Design review of the part built by this model. Coordinates are the model's own, in mm. Face numbers are marked on the shaded views. A direction names the side the tool comes from. Give positions to 0.01 mm unless a question says otherwise; leave off trailing zeros. Loops run counter-clockwise (first coordinate to the right, second up) from the corner with the lowest first, then second, coordinate; pieces in that order, holes last. Notation, with made-up numbers: (41.5, -4.5) -> (59.5, -4.5) arc R33 cw to (59.5, 27.5) -> close; hole circle Ø2 at (59, 41.5). An arc over 180 degrees is marked (long way). Answer in a Markdown table with one row per item. Add a question column.
(1) Draft analysis for pull direction X (two halves, no side actions). For the marked faces 4, 5 and 6, state which applies: +X half, -X half, draft (parallel to the pull), parting line (faces both ways), or undercut.
(2) For pin 1 (0.8 mm diameter, centred on y = -1, z = -1.5, fed in from +X), flat-tipped, find the tip position at first contact; note if it passes through.
(3) Consider section D-D on z = -2. Write out the cut boundary in (x, y), then the cut area to 3 significant figures.
(4) Consider section B-B on y = -1.15. Write out the cut boundary in (x, z), then the cut area to 3 significant figures.
(5) Consider section A-A on x = -6. Write out the cut boundary in (y, z).
(6) For the marked faces 1, 2 and 3, list the 3-axis set-ups (+Z, -Z, +X, -X, +Y, -Y) from which the entire face can be reached by the end or side of a thin tool; tool diameter is ignored.
(7) Consider section C-C on x = -1.25. Write out the cut boundary in (y, z), then the cut area to 3 significant figures.
(8) For line 1 (Y direction, x = -0.25, z = -1.7); line 2 (X direction, y = -1.4, z = -1.25); line 3 (Z direction, x = -6, y = -1.45), list the stretches that pass through material, from the lowest coordinate up.
from build123d import *

# Parameters (mm, degrees)
F0_R      = 0.5
F1_DEPTH  = 2
F0_R_2    = 0.4
F2_DEPTH  = 0.5
F3_R      = 0.4
F4_DEPTH  = 0.5
F5_D      = 1
F6_DEPTH  = 0.5
F7_DEPTH  = 0.5
F8_R      = 0.3
F9_W      = 2
F9_H      = 0.1
F10_DEPTH = 25
F11_R     = 0.49999


# Not quite as in the source:
# - a fillet or chamfer is up to 0.001 mm smaller than in the source, because OpenCascade refuses the exact size
# - a feature names something its author has since deleted; it is built from what else it names


with BuildPart() as f1:
    # F0 (on Front) → F1 (new body)
    with BuildSketch(Plane.XZ):
        with BuildLine():
            Line((-1.5, -1.2454767711), (-1.5, -0.24940907))
            Line((-1.5, -0.24940907), (-4, -0.24940907))
            ThreePointArc((-4, -0.24940907), (-5, -1.24940907), (-4, -2.24940907))
            Line((-4, -2.24940907), (-1.5, -2.24940907))
            Line((-1.5, -2.24940907), (-1.5, -1.2454767711))
        make_face()
        with BuildLine():
            ThreePointArc((-4, -2.24940907), (-5, -1.24940907), (-4, -0.24940907))
            Line((-4, -0.24940907), (-7, -0.24940907))
            Line((-7, -0.24940907), (-7, -2.24940907))
            Line((-7, -2.24940907), (-4, -2.24940907))
        make_face()
        with Locations((-6, -1.24940907)):
            Circle(F0_R, mode=Mode.SUBTRACT)
        with Locations((-6, -1.24940907)):
            Circle(F0_R)
    extrude(amount=F1_DEPTH)

    # F0 (on Front) → F2 (join)
    with BuildSketch(Plane.XZ):
        with BuildLine():
            Line((-1.5, -1.2454767711), (-1.5, -0.24940907))
            Line((-1.5, -0.24940907), (-4, -0.24940907))
            ThreePointArc((-4, -0.24940907), (-5, -1.24940907), (-4, -2.24940907))
            Line((-4, -2.24940907), (-1.5, -2.24940907))
            Line((-1.5, -2.24940907), (-1.5, -1.2454767711))
        make_face()
        with BuildLine():
            Line((0, -0.24940907), (-1, -0.24940907))
            Line((-1, -0.24940907), (-1, -2.24940907))
            Line((-1, -2.24940907), (0, -2.24940907))
            ThreePointArc((0, -2.24940907), (1, -1.24940907), (0, -0.24940907))
        make_face()
        with Locations((0, -1.24940907)):
            Circle(F0_R_2, mode=Mode.SUBTRACT)
        Polygon((-1, -2.24940907), (-1, -0.24940907), (-1.5, -0.24940907), (-1.5, -1.2454767711), (-1.5, -2.24940907), align=None)
        with Locations((0, -1.24940907)):
            Circle(F0_R_2)
    extrude(amount=-F2_DEPTH)

    # F3 (on face) → F4 (join)
    with BuildSketch(Plane.XZ.offset(2)):
        with BuildLine():
            Line((-1.5, -2.24940907), (-1.5, -0.24940907))
            Line((-1.5, -0.24940907), (-4, -0.24940907))
            ThreePointArc((-4, -0.24940907), (-5, -1.24940907), (-4, -2.24940907))
            Line((-4, -2.24940907), (-1.5, -2.24940907))
        make_face()
        with BuildLine():
            Line((0, -0.24940907), (-1, -0.24940907))
            Line((-1, -0.24940907), (-1.5, -0.24940907))
            Line((-1.5, -0.24940907), (-1.5, -2.24940907))
            Line((-1.5, -2.24940907), (0, -2.24940907))
            ThreePointArc((0, -2.24940907), (1, -1.24940907), (0, -0.24940907))
        make_face()
        with Locations((0, -1.24940907)):
            Circle(F3_R, mode=Mode.SUBTRACT)
        with Locations((0, -1.24940907)):
            Circle(F3_R)
    extrude(amount=F4_DEPTH)

    # F5 (through all)
    with Locations(Plane(origin=(0, 0, 0), x_dir=(1, 0, 0), z_dir=(0, 1, 0))):
        with Locations((-6, 1.24940907)):
            Hole(F5_D / 2)

    # F0 (on Front) → F6 (join)
    with BuildSketch(Plane.XZ):
        with Locations((0, -1.24940907)):
            Circle(F0_R_2)
    extrude(amount=F6_DEPTH)

    # F3 (on face) → F7 (join)
    with BuildSketch(Plane.XZ.offset(2)):
        with Locations((0, -1.24940907)):
            Circle(F3_R)
    extrude(amount=-F7_DEPTH)

    # F8
    f8_edges = [f1.edges().sort_by_distance(p)[0] for p in [
        (-0.4, -0.5, -1.249409),
        (-0.4, -1.5, -1.249409),
    ]]
    fillet(f8_edges, radius=F8_R)

    # F9 (on face) → F10 (cut)
    with BuildSketch(Plane(origin=(0, 0, -2.24940907), x_dir=(1, 0, 0), z_dir=(0, 0, -1))):
        with Locations((-6, 1.95)):
            Rectangle(F9_W, F9_H)
        with Locations((-6, 0.05)):
            Rectangle(F9_W, F9_H)
    extrude(amount=-F10_DEPTH, mode=Mode.SUBTRACT)

    # F11 (radius 0.5 in the source; OpenCascade refuses exactly that, so slightly less here)
    f11_edges = [f1.edges().sort_by_distance(p)[0] for p in [
        (-7, -1.9, -1.249409),
        (-7, -0.1, -1.249409),
        (-1.5, -1, -0.249409),
        (-1.5, -1, -2.249409),
    ]]
    fillet(f11_edges, radius=F11_R)


solid = f1.part
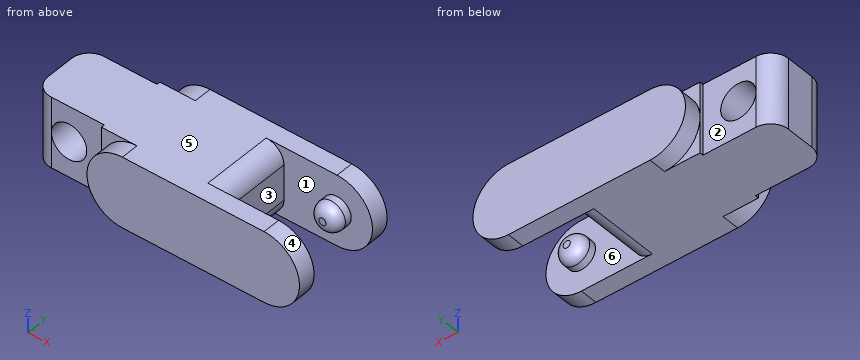
Values follow:
| question | item | result |
|---|---|---|
| 1 | face 4 | +X half |
| 1 | face 5 | draft |
| 1 | face 6 | undercut |
| 2 | pin 1 | x = -1.5 |
| 3 | outline | (-7, -1.4) arc R0.5 ccw to (-6.5, -1.9) -> (-5, -1.9) -> (-5, -2) -> (-4.66, -2) -> (-4.66, -2.5) -> (0.66, -2.5) -> (0.66, -2) -> (-1.57, -2) -> (-1.57, 0) -> (0.66, 0) -> (0.66, 0.5) -> (-4.66, 0.5) -> (-4.66, 0) -> (-5, 0) -> (-5, -0.1) -> (-6.5, -0.1) arc R0.5 ccw to (-7, -0.6) -> close |
| 3 | area | 15.7 mm2 |
| 4 | outline | (-7, -2.25) -> (-2, -2.25) arc R0.5 ccw to (-1.5, -1.75) -> (-1.5, -0.75) arc R0.5 ccw to (-2, -0.25) -> (-7, -0.25) -> close; hole circle Ø1 at (-6, -1.25) |
| 4 | area | 10.1 mm2 |
| 5 | outline | (-1.9, -2.25) -> (-0.1, -2.25) -> (-0.1, -1.75) -> (-1.9, -1.75) -> close; (-1.9, -0.75) -> (-0.1, -0.75) -> (-0.1, -0.25) -> (-1.9, -0.25) -> close |
| 6 | face 1 | none |
| 6 | face 2 | +Z, -Z, -X, +Y |
| 6 | face 3 | +Z, -Z |
| 7 | outline | (-2.5, -2.25) -> (-2, -2.25) -> (-2, -0.25) -> (-2.5, -0.25) -> close; (0, -2.25) -> (0.5, -2.25) -> (0.5, -0.25) -> (0, -0.25) -> close |
| 7 | area | 2.00 mm2 |
| 8 | line 1 | -2.5 to -2, 0 to 0.5 |
| 8 | line 2 | -7 to -6.5, -5.5 to -1.5 |
| 8 | line 3 | -2.25 to -1.75, -0.75 to -0.25 |
